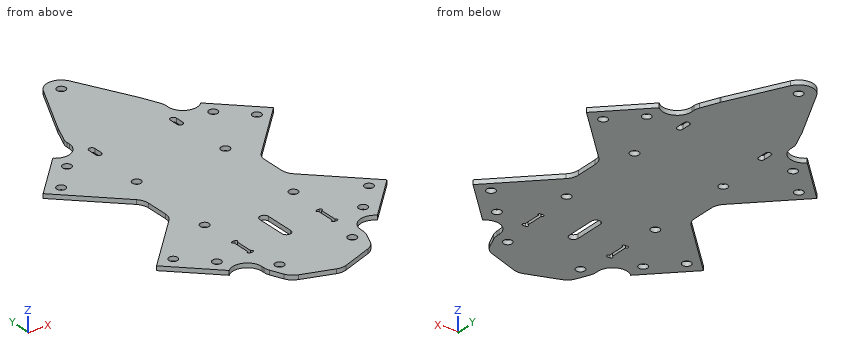
```python
from build123d import *

# Parameters (mm, degrees)
F0_R        = 1.5
F1_DEPTH    = 1.5
F2_T1_DEPTH = 1.5
F3_T1_DEPTH = 1.5
F3_T3_DEPTH = 6.6314425489
F3_T5_DEPTH = 12.4086164325
F3_T7_DEPTH = 10.4285714286
F3_T9_DEPTH = 2.253003807
F5_DEPTH    = 25


# Not quite as in the source:
# - a fillet or chamfer that OpenCascade refuses, or shapes differently, is made with other operations: its cross-section is extruded or revolved along the edge and cut away or added


with BuildPart() as f1:
    # F0 (on Top) → F1 (new body)
    with BuildSketch(Plane.XY):
        with BuildLine():
            Line((-25.4558441227, 39.5979797464), (-39.5979797464, 25.4558441227))
            Line((-39.5979797464, 25.4558441227), (-20, 5.8578643763))
            Line((-20, 5.8578643763), (-20, -5.8578643763))
            Line((-20, -5.8578643763), (-39.5979797464, -25.4558441227))
            Line((-39.5979797464, -25.4558441227), (-25.4558441227, -39.5979797464))
            Line((-25.4558441227, -39.5979797464), (-17, -31.1421356237))
            Line((-17, -31.1421356237), (-17, -45.25))
            Line((-17, -45.25), (-14, -52.25))
            Line((-14, -52.25), (0, -57.25))
            Line((0, -57.25), (14, -52.25))
            Line((14, -52.25), (17, -45.25))
            Line((17, -45.25), (17, -31.1421356237))
            Line((17, -31.1421356237), (25.4558441227, -39.5979797464))
            Line((25.4558441227, -39.5979797464), (39.5979797464, -25.4558441227))
            Line((39.5979797464, -25.4558441227), (20, -5.8578643763))
            Line((20, -5.8578643763), (20, 5.8578643763))
            Line((20, 5.8578643763), (39.5979797464, 25.4558441227))
            Line((39.5979797464, 25.4558441227), (25.4558441227, 39.5979797464))
            Line((25.4558441227, 39.5979797464), (17, 31.1421356237))
            Line((17, 31.1421356237), (17, 45.25))
            Line((17, 45.25), (14, 52.25))
            Line((14, 52.25), (4.468852459, 71.2426229508))
            ThreePointArc((4.468852459, 71.2426229508), (0, 74), (-4.468852459, 71.2426229508))
            Line((-4.468852459, 71.2426229508), (-14, 52.25))
            Line((-14, 52.25), (-17, 45.25))
            Line((-17, 45.25), (-17, 31.1421356237))
            Line((-17, 31.1421356237), (-25.4558441227, 39.5979797464))
        make_face()
        with Locations((-33.6347763109, -25.1494949366)):
            Circle(F0_R, mode=Mode.SUBTRACT)
        with Locations((-25.1494949366, -33.6347763109)):
            Circle(F0_R, mode=Mode.SUBTRACT)
        with Locations((-12.5, -45.25)):
            Circle(F0_R, mode=Mode.SUBTRACT)
        with BuildLine():
            ThreePointArc((-1.5, -22), (0, -20.5), (1.5, -22))
            Line((1.5, -22), (1.5, -32))
            ThreePointArc((1.5, -32), (0, -33.5), (-1.5, -32))
            Line((-1.5, -32), (-1.5, -22))
        make_face(mode=Mode.SUBTRACT)
        with Locations((-15.25, -15.25)):
            Circle(F0_R, mode=Mode.SUBTRACT)
        with Locations((12.5, -45.25)):
            Circle(F0_R, mode=Mode.SUBTRACT)
        with Locations((25.1494949366, -33.6347763109)):
            Circle(F0_R, mode=Mode.SUBTRACT)
        with Locations((33.6347763109, -25.1494949366)):
            Circle(F0_R, mode=Mode.SUBTRACT)
        with Locations((15.25, -15.25)):
            Circle(F0_R, mode=Mode.SUBTRACT)
        with Locations((-33.6347763109, 25.1494949366)):
            Circle(F0_R, mode=Mode.SUBTRACT)
        with Locations((-25.1494949366, 33.6347763109)):
            Circle(F0_R, mode=Mode.SUBTRACT)
        with Locations((-15.25, 15.25)):
            Circle(F0_R, mode=Mode.SUBTRACT)
        with BuildLine():
            Line((-15, 34), (-15, 37))
            ThreePointArc((-15, 37), (-14, 38), (-13, 37))
            Line((-13, 37), (-13, 34))
            ThreePointArc((-13, 34), (-14, 33), (-15, 34))
        make_face(mode=Mode.SUBTRACT)
        with Locations((0, 69)):
            Circle(F0_R, mode=Mode.SUBTRACT)
        with Locations((15.25, 15.25)):
            Circle(F0_R, mode=Mode.SUBTRACT)
        with BuildLine():
            ThreePointArc((13, 37), (14, 38), (15, 37))
            Line((15, 37), (15, 34))
            ThreePointArc((15, 34), (14, 33), (13, 34))
            Line((13, 34), (13, 37))
        make_face(mode=Mode.SUBTRACT)
        with Locations((25.1494949366, 33.6347763109)):
            Circle(F0_R, mode=Mode.SUBTRACT)
        with Locations((33.6347763109, 25.1494949366)):
            Circle(F0_R, mode=Mode.SUBTRACT)
    extrude(amount=F1_DEPTH)

    # F2: fillet of radius 5 on 4 edges, made by hand

    # F2_s2 → F2_t1 (join)
    with BuildSketch(Plane.XY):
        with BuildLine():
            ThreePointArc((17, -43.2114464198), (20.0352125578, -38.613663225), (25.4558441227, -39.5979797464))
            Line((25.4558441227, -39.5979797464), (17, -31.1421356237))
            Line((17, -31.1421356237), (17, -43.2114464198))
        make_face()
        with BuildLine():
            ThreePointArc((-25.4558441227, -39.5979797464), (-20.0352125578, -38.613663225), (-17, -43.2114464198))
            Line((-17, -43.2114464198), (-17, -31.1421356237))
            Line((-17, -31.1421356237), (-25.4558441227, -39.5979797464))
        make_face()
        with BuildLine():
            ThreePointArc((-17, 43.2114464198), (-20.0352125578, 38.613663225), (-25.4558441227, 39.5979797464))
            Line((-25.4558441227, 39.5979797464), (-17, 31.1421356237))
            Line((-17, 31.1421356237), (-17, 43.2114464198))
        make_face()
        with BuildLine():
            ThreePointArc((25.4558441227, 39.5979797464), (20.0352125578, 38.613663225), (17, 43.2114464198))
            Line((17, 43.2114464198), (17, 31.1421356237))
            Line((17, 31.1421356237), (25.4558441227, 39.5979797464))
        make_face()
    extrude(amount=F2_T1_DEPTH)

    # F3: fillet of radius 5 on 13 edges, made by hand

    # F3_s2 → F3_t1 (join)
    with BuildSketch(Plane.XY):
        with BuildLine():
            ThreePointArc((20, 3.7867965644), (20.3806023374, 5.7002137262), (21.4644660941, 7.3223304703))
            Line((21.4644660941, 7.3223304703), (20, 5.8578643763))
            Line((20, 5.8578643763), (20, 3.7867965644))
        make_face()
        with BuildLine():
            ThreePointArc((21.4644660941, -7.3223304703), (20.3806023374, -5.7002137262), (20, -3.7867965644))
            Line((20, -3.7867965644), (20, -5.8578643763))
            Line((20, -5.8578643763), (21.4644660941, -7.3223304703))
        make_face()
        with BuildLine():
            ThreePointArc((-20, -3.7867965644), (-20.3806023374, -5.7002137262), (-21.4644660941, -7.3223304703))
            Line((-21.4644660941, -7.3223304703), (-20, -5.8578643763))
            Line((-20, -5.8578643763), (-20, -3.7867965644))
        make_face()
        with BuildLine():
            ThreePointArc((-21.4644660941, 7.3223304703), (-20.3806023374, 5.7002137262), (-20, 3.7867965644))
            Line((-20, 3.7867965644), (-20, 5.8578643763))
            Line((-20, 5.8578643763), (-21.4644660941, 7.3223304703))
        make_face()
    extrude(amount=F3_T1_DEPTH)

    # F3_s4 → F3_t3 (cut)
    with BuildSketch(Plane.XY.offset(-2.5657212744)):
        with BuildLine():
            ThreePointArc((16.5957251501, -46.1933079831), (16.897888614, -45.2290408516), (17, -44.2237114902))
            Line((17, -44.2237114902), (17, -45.25))
            Line((17, -45.25), (16.5957251501, -46.1933079831))
        make_face()
        with BuildLine():
            ThreePointArc((-17, -44.2237114902), (-16.897888614, -45.2290408516), (-16.5957251501, -46.1933079831))
            Line((-16.5957251501, -46.1933079831), (-17, -45.25))
            Line((-17, -45.25), (-17, -44.2237114902))
        make_face()
        with BuildLine():
            ThreePointArc((-17, 44.2237114902), (-16.897888614, 45.2290408516), (-16.5957251501, 46.1933079831))
            Line((-16.5957251501, 46.1933079831), (-17, 45.25))
            Line((-17, 45.25), (-17, 44.2237114902))
        make_face()
        with BuildLine():
            ThreePointArc((17, 44.2237114902), (16.897888614, 45.2290408516), (16.5957251501, 46.1933079831))
            Line((16.5957251501, 46.1933079831), (17, 45.25))
            Line((17, 45.25), (17, 44.2237114902))
        make_face()
    extrude(amount=F3_T3_DEPTH, mode=Mode.SUBTRACT)

    # F3_s6 → F3_t5 (cut)
    with BuildSketch(Plane.XY.offset(-5.4543082162)):
        with BuildLine():
            ThreePointArc((11.9453797416, -52.9837929494), (13.6881897161, -51.9182763344), (14.8594229067, -50.2446798843))
            Line((14.8594229067, -50.2446798843), (14, -52.25))
            Line((14, -52.25), (11.9453797416, -52.9837929494))
        make_face()
        with BuildLine():
            ThreePointArc((-14.8594229067, -50.2446798843), (-13.6881897161, -51.9182763344), (-11.9453797416, -52.9837929494))
            Line((-11.9453797416, -52.9837929494), (-14, -52.25))
            Line((-14, -52.25), (-14.8594229067, -50.2446798843))
        make_face()
    extrude(amount=F3_T5_DEPTH, mode=Mode.SUBTRACT)

    # F3_s8 → F3_t7 (cut)
    with BuildSketch(Plane.XY.offset(-4.4642857143)):
        with BuildLine():
            ThreePointArc((-1.681681985, -56.6493992911), (0, -56.9406897331), (1.681681985, -56.6493992911))
            Line((1.681681985, -56.6493992911), (0, -57.25))
            Line((0, -57.25), (-1.681681985, -56.6493992911))
        make_face()
    extrude(amount=F3_T7_DEPTH, mode=Mode.SUBTRACT)

    # F3_s10 → F3_t9 (cut)
    with BuildSketch(Plane.XY.offset(-0.3765019035)):
        with BuildLine():
            ThreePointArc((-13.9324518552, 52.3846025166), (-13.9979436343, 52.2490444272), (-14.0593245463, 52.1115760587))
            Line((-14.0593245463, 52.1115760587), (-14, 52.25))
            Line((-14, 52.25), (-13.9324518552, 52.3846025166))
        make_face()
        with BuildLine():
            ThreePointArc((14.0593245463, 52.1115760587), (13.9979436343, 52.2490444272), (13.9324518552, 52.3846025166))
            Line((13.9324518552, 52.3846025166), (14, 52.25))
            Line((14, 52.25), (14.0593245463, 52.1115760587))
        make_face()
    extrude(amount=F3_T9_DEPTH, mode=Mode.SUBTRACT)

    # F4 (on face) → F5 (cut)
    with BuildSketch(Plane.XY.offset(1.5)):
        with BuildLine():
            Line((-14, -27.25), (-15, -27.25))
            ThreePointArc((-15, -27.25), (-15.5, -27.75), (-15, -28.25))
            Line((-15, -28.25), (-15, -34.25))
            ThreePointArc((-15, -34.25), (-15.5, -34.75), (-15, -35.25))
            Line((-15, -35.25), (-14, -35.25))
            ThreePointArc((-14, -35.25), (-13.5, -34.75), (-14, -34.25))
            Line((-14, -34.25), (-14, -28.25))
            ThreePointArc((-14, -28.25), (-13.5, -27.75), (-14, -27.25))
        make_face()
        with BuildLine():
            ThreePointArc((15, -28.25), (15.5, -27.75), (15, -27.25))
            Line((15, -27.25), (14, -27.25))
            ThreePointArc((14, -27.25), (13.5, -27.75), (14, -28.25))
            Line((14, -28.25), (14, -34.25))
            ThreePointArc((14, -34.25), (13.5, -34.75), (14, -35.25))
            Line((14, -35.25), (15, -35.25))
            ThreePointArc((15, -35.25), (15.5, -34.75), (15, -34.25))
            Line((15, -34.25), (15, -28.25))
        make_face()
    extrude(amount=-F5_DEPTH, mode=Mode.SUBTRACT)


solid = f1.part
```
Geometry check sheet. Reference: the model listing, model coordinates, mm. Round coordinates to 2 decimals unless told otherwise and drop trailing zeros. Order: outer loops, then holes, each group sorted by start corner. A loop starts at its lowest first (then second) coordinate and runs counter-clockwise, first axis right, second up. Notation, with made-up numbers: (5.25, -10.75) - (60.25, -10.75) arc R20 ccw to (60.25, 26.25) - close; hole circle Ø6 at (53, 56.25). An arc over 180 degrees is marked (long way). Use a Markdown table: item, result. Add a question column.
(1) Sectioned sample at A-A, the plane y = -9.5. Enter the section's corners in (x, z).
(2) Sectioned sample at B-B, the plane z = 1.05. Count the separate pieces of the cut face and the enclosed holes in it, and give its area (3 significant figures).
(3) Sectioned sample at C-C, the plane x = -9.5. Enter the section's corners in (y, z), and give its area (3 significant figures).
(4) Depth check by flat-ended pin: pin 1 (0.8 mm diameter, centred on y = -32, z = 0.5, fed in from -X); pin 2 (0.8 mm diameter, centred on y = 44, z = 0.5, fed in from +X); pin 3 (0.5 mm diameter, centred on y = 44, z = 1, fed in from -X). Enter the tip coordinate at first touch or a pass-through.
(5) Material ranges on line 1 along Y through (x, z) = (24.5, 0.1); line 2 along X through (y, z) = (-26.5, 1); line 3 along Y through (x, z) = (15.25, 0.55), recorded low to high. Write a range as [from, to].
Answers below:
| question | item | result |
|---|---|---|
| 1 | outline | (-23.64, 0) - (23.64, 0) - (23.64, 1.5) - (-23.64, 1.5) - close |
| 2 | separate pieces | 1 |
| 2 | enclosed holes | 20 |
| 2 | area | 5,700 mm² |
| 3 | outline | (-53.86, 0) - (61.22, 0) - (61.22, 1.5) - (-53.86, 1.5) - close |
| 3 | area | 173 mm² |
| 4 | pin 1 | x = -33.45 |
| 4 | pin 2 | x = 17 |
| 4 | pin 3 | x = -17 |
| 5 | line 1 | [-38.88, -34.99], [-32.28, -10.36], [10.36, 32.28], [34.99, 38.88] |
| 5 | line 2 | [-38.55, -34.29], [-32.98, -1.5], [1.5, 32.98], [34.29, 38.55] |
| 5 | line 3 | [-49.33, -35.18], [-34.32, -28.18], [-27.32, -16.75], [-13.75, 13.75], [16.75, 49.33] |
